```python
from build123d import *

# Parameters (mm, degrees)
BOSS_EXTRUDE1_DEPTH = 5
FILLET1_R           = 3
SKETCH2_R           = 2
CUT_EXTRUDE1_DEPTH  = 7
SKETCH3_R           = 2
CUT_EXTRUDE2_DEPTH  = 7


with BuildPart() as part:
    # Sketch1 → Boss-Extrude1 (new, symmetric)
    with BuildSketch(Plane.XY):
        with BuildLine():
            Line((24.49935999, -21), (32.49935999, -21))
            Line((32.49935999, -21), (32.49935999, 11))
            Line((32.49935999, 11), (24.49935999, 11))
            ThreePointArc((24.49935999, 11), (10.203242171, 7.348405073), (-4.50064001, 6.12))
            ThreePointArc((-4.50064001, 6.12), (-16.964475696, 10.248068768), (-24.5, 21))
            Line((-24.5, 21), (-32.5, 21))
            Line((-32.5, 21), (-32.5, -11))
            Line((-32.5, -11), (-24.5, -11))
            ThreePointArc((-24.5, -11), (-10.203882181, -7.348405073), (4.5, -6.12))
            ThreePointArc((4.5, -6.12), (16.963835686, -10.248068768), (24.49935999, -21))
        make_face()
    extrude(amount=BOSS_EXTRUDE1_DEPTH, both=True)

    # Fillet1
    fillet1_edges = [part.edges().sort_by_distance(p)[0] for p in [
        (28.49935999, -21, -5),
        (16.963835686, -10.248068768, -5),
        (-10.203882181, -7.348405073, -5),
        (-28.5, -11, -5),
        (-28.5, 21, -5),
        (-16.964475696, 10.248068768, -5),
        (10.203242171, 7.348405073, 5),
        (10.203242171, 7.348405073, -5),
        (28.49935999, 11, -5),
        (-16.964475696, 10.248068768, 5),
        (-28.5, 21, 5),
        (-28.5, -11, 5),
        (-10.203882181, -7.348405073, 5),
        (16.963835686, -10.248068768, 5),
        (28.49935999, -21, 5),
        (28.49935999, 11, 5),
    ]]
    fillet(fillet1_edges, radius=FILLET1_R)

    # Sketch2 → Cut-Extrude1 (cut)
    with BuildSketch(Plane(origin=(32.49935999, 0, 0), x_dir=(0, 0, -1), z_dir=(1, 0, 0))):
        with Locations((0, -13)):
            Circle(SKETCH2_R)
        with Locations((0, 3)):
            Circle(SKETCH2_R)
    extrude(amount=-CUT_EXTRUDE1_DEPTH, mode=Mode.SUBTRACT)

    # Sketch3 → Cut-Extrude2 (cut)
    with BuildSketch(Plane.ZY.offset(32.5)):
        with Locations(Location((0, 13, 0), (0, 0, 270))):
            Circle(SKETCH3_R)
        with Locations(Location((0, -3, 0), (0, 0, 270))):
            Circle(SKETCH3_R)
    extrude(amount=-CUT_EXTRUDE2_DEPTH, mode=Mode.SUBTRACT)


solid = part.part
```
Can you work these out from the model? Positions are in its coordinate system, mm. A direction names the side the tool comes from. Round coordinates to 2 decimals unless told otherwise and drop trailing zeros. Loops run counter-clockwise (first coordinate to the right, second up) from the corner with the lowest first, then second, coordinate; pieces in that order, holes last. Notation, with made-up numbers: M 12.25,50.25 L 23.25,50.25 A24 cw 23.25,74.25 Z; hole C 54,-15 d10. An arc over 180 degrees is marked long. Answer in a Markdown table with one row per item.
1. If we section it at A-A, the plane z = 0: Please give me the cut outline in (x, y).
Established:
| item | result |
|---|---|
| outline | M -32.5,-11 L -24.5,-11 A88.6 cw 4.5,-6.12 A20.88 cw 24.5,-21 L 32.5,-21 L 32.5,-15 L 25.5,-15 L 25.5,-11 L 32.5,-11 L 32.5,1 L 25.5,1 L 25.5,5 L 32.5,5 L 32.5,11 L 24.5,11 A88.6 cw -4.5,6.12 A20.88 cw -24.5,21 L -32.5,21 L -32.5,15 L -25.5,15 L -25.5,11 L -32.5,11 L -32.5,-1 L -25.5,-1 L -25.5,-5 L -32.5,-5 Z |
2. On a 3-axis mill with a long thin cutter (end or side, diameter ignored), from which of +Z, -Z, +X, -X, +Y, -Y can I reach the whole of each face in a straight line? I mean faces 1 (the face through (-25.5, 13, 0)), 2 (the face through (-28.44, -10.14, 4.1)), 3 (the face through (-16.814, 10.137, 0.028)). Say none if no direction works.
Established:
| item | result |
|---|---|
| face 1 | -X |
| face 2 | +Z, -X, -Y |
| face 3 | +Z, -Z, +Y |
3. Please list where these lines run through material, in increasing order: line 1 (Y direction, x = 30.25, z = 0); line 2 (Z direction, x = -29, y = -3); line 3 (Y direction, x = -2, z = -3.25). Write a range as from..to.
Established:
| item | result |
|---|---|
| line 1 | -21..-15, -11..1, 5..11 |
| line 2 | -5..-2, 2..5 |
| line 3 | -6.09..5.88 |
4. I'm going to push flat-ended pins straight in: pin 1 Ø4 at (x, z) = (-17.5, 1.5) entering from -Y; pin 2 Ø3 at (y, z) = (13, 0) entering from +X; pin 3 Ø2 at (x, z) = (-26.5, 0.5) entering from -Y. Where does each tip first touch, or does it pass through?
Established:
| item | result |
|---|---|
| pin 1 | y = -9.43 |
| pin 2 | x = -18.49 |
| pin 3 | y = -11 |
5. Thinking about a two-plate mould opening in X: for faces 4 (the face through (-25.5, -3, 0)), 5 (the face through (-29, -11, 0)), 6 (the face through (10.407, 7.383, 0.028)), which applies, pulls with the +X half, pulls with the -X half, needs draft (parallel to the pull), parting line crosses it, or undercut?
Established:
| item | result |
|---|---|
| face 4 | pulls with the -X half |
| face 5 | needs draft |
| face 6 | undercut |
6. If we section it at B-B, the plane z = -3.5: Please give me the cut outline in (x, y), plus the area to 3 significant figures.
Established:
| item | result |
|---|---|
| outline | M -32.5,-10.6 L -24.57,-10.6 A89 cw 4.5,-5.72 A21.28 cw 24.8,-20.6 L 32.5,-20.6 L 32.5,10.6 L 24.57,10.6 A89 cw -4.5,5.72 A21.28 cw -24.8,20.6 L -32.5,20.6 Z |
| area | 1,300 mm² |
